Autodesk Fusion 360 part; units mm, degrees
sketch "Sketch1" plane through (0, 0, 0) normal (0, 0, 1) x (1, 0, 0)
  line L0 (0, 0) -> (40, 0)
  line L1 (40, 0) -> (40, 28)
  line L2 (40, 28) -> (0, 28)
  line L3 (0, 28) -> (0, 0)
  line L4 (0, 0) -> (40, 0) construction
  line L5 (40, 0) -> (40, 20) construction
  line L6 (40, 20) -> (0, 20) construction
  line L7 (0, 20) -> (0, 0) construction
  line L8 (0, 20) -> (20, 20) construction
  line L9 (20, 20) -> (20, 0) construction
  line L10 (20, 0) -> (0, 0) construction
  line L11 (0, 0) -> (0, 20) construction
  line L12 (0, 0) -> (20, 20) construction
  line L13 (0, 20) -> (20, 0) construction
  line L14 (20, 20) -> (40, 0) construction
  line L15 (20, 0) -> (40, 20) construction
  circle A0 centre (10, 10) radius 5
  circle A1 centre (30, 10) radius 5
  dimension "d1" = 40
  dimension "d2" = 28
  dimension "d3" = 20
  dimension "d4" = 10
  dimension "d5" = 10
extrude "Extrude1" add sketch "Sketch1" against normal blind 3
sketch "Sketch2" plane through (0, 0, -3) normal (0, 0, -1) x (1, 0, 0)
  circle A0 centre (10, -10) radius 5
  circle A1 centre (30, -10) radius 5
  line L0 (0, 0) -> (0, -28)
  line L1 (0, -28) -> (40, -28)
  line L2 (40, -28) -> (40, 0)
  line L3 (40, 0) -> (0, 0)
  circle A2 centre (30, -10) radius 2.75
  circle A3 centre (10, -10) radius 2.75
  dimension "d8" = 5.5
  dimension "d9" = 5.5
extrude "Extrude2" add sketch "Sketch2" along normal blind 5 contours A0 | A1 | L0 L1 L2 L3
chamfer "Chamfer1" distance 8 angle 45 1 edges at (0, 28, -4)
chamfer "Chamfer2" distance 8 angle 45 1 edges at (40, 28, -4)
chamfer "Chamfer3" distance 0.5 angle 45 8 edges at (4, 24, 0) (0, 10, 0) (20, 0, 0) (40, 10, 0) (36, 24, 0) (20, 28, 0) (5.3384, 11.8081, 0) (25.3384, 11.8081, 0)
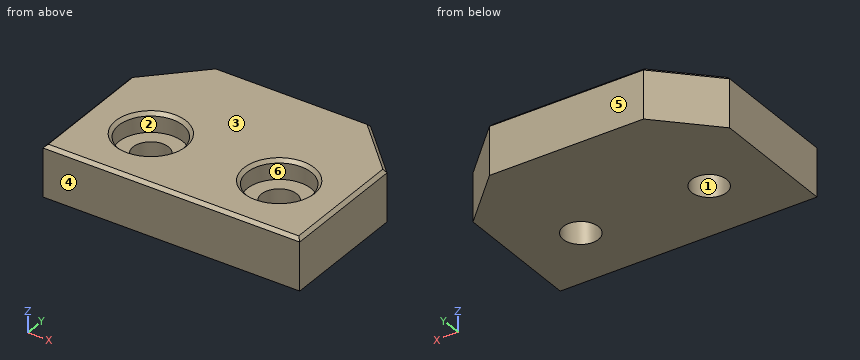
Here's how the part is built. I have some questions about the finished solid (model axes, mm). Face numbers are marked on the shaded views. A direction names the side the tool comes from. Round coordinates to 2 decimals unless told otherwise and drop trailing zeros. Write each loop counter-clockwise with the first axis right and the second up, starting at its lowest first coordinate (ties: lowest second). Pieces come first, ordered by that corner, then holes.
Q1. If we section it at D-D on z = -1.5: Write out the boundary of the cut face in (x, y).
Q2. Which directions (+Z, -Z, +X, -X, +Y, -Y) give clear straight access to the entire face, cutting with the end or side of a thin tool? Please do the marked faces 1 and 2.
Q3. If we section it at B-B on z = -5.5: Write out the boundary of the cut face in (x, y), plus the area to 3 significant figures.
Q4. If we mould it in two halves opening along Y, with no side actions, what happens to the marked faces 3, 4, 5 and 6? For each: +Y half, -Y half, draft (parallel to the pull), parting line (faces both ways), or undercut.
Q5. Will this pin go through, and if not, where does the flat tip stop? P1, Ø3, axis at x = 9.5, y = 8, coming from the +Z side.
Q6. Please list where these lines run through material, in increasing order: probe 1 along X at (y, z) = (10, -6.75); probe 2 along X at (y, z) = (8.25, -3.5); probe 3 along Y at (x, z) = (30, -2.25).
Q7. If we section it at C-C on x = 30: Write out the boundary of the cut face in (y, z), plus the area to 3 significant figures.
Q8. If we section it at A-A on y = 10: Write out the boundary of the cut face in (x, z), plus the area to 3 significant figures.
Answer below:
1. outline: (0, 0) - (40, 0) - (40, 20) - (32, 28) - (8, 28) - (0, 20) - close; hole circle Ø10 at (10, 10); hole circle Ø10 at (30, 10)
2. face 1: +Z, -Z
2. face 2: +Z
3. outline: (0, 0) - (40, 0) - (40, 20) - (32, 28) - (8, 28) - (0, 20) - close; hole circle Ø5.5 at (10, 10); hole circle Ø5.5 at (30, 10)
3. area: 1,010 mm2
4. face 3: draft
4. face 4: -Y half
4. face 5: +Y half
4. face 6: undercut
5. P1: stops at z = -3
6. probe 1: x = 0 to 7.25, 12.75 to 27.25, 32.75 to 40
6. probe 2: x = 0 to 7.88, 12.12 to 27.88, 32.12 to 40
6. probe 3: y = 0 to 5, 15 to 28
7. outline: (0, -8) - (7.25, -8) - (7.25, -3) - (5, -3) - (5, -0.5) - (4.5, 0) - (0.5, 0) - (0, -0.5) - close; (12.75, -8) - (28, -8) - (28, -0.5) - (27.5, 0) - (15.5, 0) - (15, -0.5) - (15, -3) - (12.75, -3) - close
7. area: 166 mm2
8. outline: (0, -8) - (7.25, -8) - (7.25, -3) - (5, -3) - (5, -0.5) - (4.5, 0) - (0.5, 0) - (0, -0.5) - close; (12.75, -8) - (27.25, -8) - (27.25, -3) - (25, -3) - (25, -0.5) - (24.5, 0) - (15.5, 0) - (15, -0.5) - (15, -3) - (12.75, -3) - close; (32.75, -8) - (40, -8) - (40, -0.5) - (39.5, 0) - (35.5, 0) - (35, -0.5) - (35, -3) - (32.75, -3) - close
8. area: 204 mm2
